from build123d import *

# Parameters (mm, degrees)
SKETCH2_R          = 11
SKETCH2_W          = 14
SKETCH2_H          = 14
CUT_EXTRUDE1_DEPTH = 8.5


with BuildPart() as part:
    # Sketch1 → Revolve1 (revolve)
    with BuildSketch(Plane.XY, mode=Mode.PRIVATE) as revolve1_sk:
        Polygon((-165, 0), (-165, 10), (10, 10), (10, 9.5), (11.5, 9.5), (11.5, 8.5), (20.5, 8.5), (20.5, 4), (21.5, 4), (21.5, 4.233), (22.267, 5), (41.733, 5), (42.5, 4.233), (42.5, 0), align=None)
    revolve(revolve1_sk.sketch.rotate(Axis((42.5, 0, 0), (-1, 0, 0)), 270), axis=Axis((42.5, 0, 0), (-1, 0, 0)))

    # Sketch2 → Cut-Extrude1 (cut)
    with BuildSketch(Plane(origin=(20.5, 0, 0), x_dir=(0, 0, -1), z_dir=(1, 0, 0))):
        Circle(SKETCH2_R)
        Rectangle(SKETCH2_W, SKETCH2_H, mode=Mode.SUBTRACT)
    extrude(amount=-CUT_EXTRUDE1_DEPTH, mode=Mode.SUBTRACT)


solid = part.part
Can you work these out from the model? Positions are in its coordinate system, mm. A direction names the side the tool comes from. Give positions to 0.01 mm unless a question says otherwise; leave off trailing zeros. Loops run counter-clockwise (first coordinate to the right, second up) from the corner with the lowest first, then second, coordinate; pieces in that order, holes last. Notation, with made-up numbers: (86, -21.5) -> (117, -21.5) arc R28 cw to (117, 14.5) -> close; hole circle Ø6 at (5.5, 22.25). An arc over 180 degrees is marked (long way). Return JSON: item names as keys, results as strings.
Q1. I want a section at C-C, the plane x = -29. List the corners of the cut face in (y, z) for me, then the cut area to 3 significant figures.
Checks:
{"outline": "circle Ø20 at (0, 0)", "area": "314 mm2"}
Q2. I want a section at A-A, the plane y = 0. List the corners of the cut face in (x, z) for me, then the cut area to 3 significant figures.
Checks:
{"outline": "(-165, -10) -> (10, -10) -> (10, -9.5) -> (11.5, -9.5) -> (11.5, -8.5) -> (12, -8.5) -> (12, -7) -> (20.5, -7) -> (20.5, -4) -> (21.5, -4) -> (21.5, -4.23) -> (22.27, -5) -> (41.73, -5) -> (42.5, -4.23) -> (42.5, 4.23) -> (41.73, 5) -> (22.27, 5) -> (21.5, 4.23) -> (21.5, 4) -> (20.5, 4) -> (20.5, 7) -> (12, 7) -> (12, 8.5) -> (11.5, 8.5) -> (11.5, 9.5) -> (10, 9.5) -> (10, 10) -> (-165, 10) -> close", "area": "3,870 mm2"}
Q3. For pin 1 Ø1.5 at (x, z) = (-34.5, -2) entering from +Y; pin 2 Ø3 at (y, z) = (1.5, -7.5) entering from +X; pin 3 Ø2 at (x, y) = (-135.5, 3) entering from -Z, each with a flat end and sliding along its axis, tell me the tip position at first contact or that it passes through.
Checks:
{"pin 1": "stops at y = 9.92", "pin 2": "stops at x = 20.5", "pin 3": "stops at z = -9.8"}
Q4. I need wall thicknesses on probe 1 along X at (y, z) = (-7.75, -0.75); probe 2 along X at (y, z) = (-4, -9); probe 3 along Y at (x, z) = (-54, 3). Which ranges of each line are inside material? Lowest first, please.
Checks:
{"probe 1": "x = -165 to 12", "probe 2": "x = -165 to 10", "probe 3": "y = -9.54 to 9.54"}
Q5. We'd pull the mould along X, two halves only. Please class faces 5 (the face through (32.14, -4.88, -1.08)), 6 (the face through (10, -4, 9)), 7 (the face through (-165, 0, 0)), 8 (the face through (20.5, -3, 3)): released by +X, released by -X, zero draft, split by the parting line, or undercut.
Checks:
{"face 5": "zero draft", "face 6": "released by +X", "face 7": "released by -X", "face 8": "undercut"}
Q6. On a 3-axis mill with a long thin cutter (end or side, diameter ignored), from which of +Z, -Z, +X, -X, +Y, -Y can I reach the whole of each face in a straight line? I mean faces 1 (the face through (16, 7, 0)), 2 (the face through (16, 0, 7)), 3 (the face through (10.76, -5.78, -7.54)), 4 (the face through (21.007, -3.905, -0.867)). Say none if no direction works.
Checks:
{"face 1": "+Z, -Z, +X, +Y", "face 2": "+Z, +X, +Y, -Y", "face 3": "+X", "face 4": "none"}
